The model under review builds one solid part; all positions refer to its coordinate system, in mm. A direction names the side the tool comes from. Round coordinates to 2 decimals unless told otherwise and drop trailing zeros. Loops run counter-clockwise (first coordinate to the right, second up) from the corner with the lowest first, then second, coordinate; pieces in that order, holes last. Notation, with made-up numbers: M -14.75,0 L 5.25,0 A15 cw 5.25,17 Z; hole C -25,51 d4. An arc over 180 degrees is marked long. Answer in a Markdown table with one row per item. Add a question column.
from build123d import *

# Parameters (mm, degrees)
SALIENTE_EXTRUIR1_DEPTH = 299.79
CROQUIS2_W              = 2
CROQUIS2_H              = 10
SALIENTE_EXTRUIR2_DEPTH = 134.79


with BuildPart() as part:
    # Croquis1 → Saliente-Extruir1 (new body)
    with BuildSketch(Plane.XY):
        Polygon((-6.5, 0), (6.5, 0), (10.956890061, 14.1), (40.206890061, 14.1), (40.206890061, -7.9), (-39.793109939, -7.9), (-39.793109939, 14.1), (-10.543109939, 14.1), align=None)
    extrude(amount=-SALIENTE_EXTRUIR1_DEPTH)

    # Croquis2 → Saliente-Extruir2 (add)
    with BuildSketch(Plane.XY):
        with Locations((-12.543109939, 19.1)):
            Rectangle(CROQUIS2_W, CROQUIS2_H)
    saliente_extruir2 = extrude(amount=-SALIENTE_EXTRUIR2_DEPTH)

    # Simetría1: Saliente-Extruir2 across plane
    add(saliente_extruir2.mirror(Plane(origin=(0, 0, 0), x_dir=(0, 0, 1), z_dir=(1, 0, 0))))


solid = part.part
1. Take a section at B-B, the plane z = -77.5. State the section outline as (x, y) points, and give its area (3 significant figures).
2. Take a section at D-D, the plane y = 6.5. State the section outline as (x, z) points.
3. Mouldability with a two-part tool opening along X and no side actions: class faces 4 (the flat face through (13.543, 19, -66)), 5 (the flat face through (1, -7.9, -148)), 6 (the flat face through (8.697, 6.951, -147.796)) as released by +X, released by -X, zero draft, split by the parting line, or undercut.
4. Take a section at A-A, the plane y = 18.5. State the section outline as (x, z) points.
5. Take a section at C-C, the plane x = 1. State the section outline as (y, z) points, and give its area (3 significant figures).
6. Machinability: for faces 1 (the flat face through (1, -2, 0)), 2 (the flat face through (0, 0, -148)), 3 (the flat face through (-13.543, 19, -66)), which of the approach directions +Z, -Z, +X, -X, +Y, -Y give a long, thin tool a straight path to every point of the face, cutting with its end or side? Answer none if there is none.
7. To check wall thickness, follow probe 1 along X at (y, z) = (20.5, -17); probe 2 along Y at (x, z) = (-18.5, -103.5); probe 3 along Y at (x, z) = (-6, -154). State the ranges of each line that lie inside material, in increasing order.
8. For pin 1 Ø4 at (x, z) = (-1, -153.5) entering from +Y; pin 2 Ø1.6 at (x, y) = (12.5, 20) entering from -Z; pin 3 Ø1 at (x, z) = (18, -82.5) entering from +Y; pin 4 Ø1 at (x, y) = (-6.5, 8.5) entering from +Z, all flat-tipped, find the tip position at first contact; note any pin that passes through.
Check sheet entries:
| question | item | result |
|---|---|---|
| 1 | outline | M -39.79,-7.9 L 40.21,-7.9 L 40.21,14.1 L 13.54,14.1 L 13.54,24.1 L 11.54,24.1 L 11.54,14.1 L 10.96,14.1 L 6.5,0 L -6.5,0 L -10.54,14.1 L -11.54,14.1 L -11.54,24.1 L -13.54,24.1 L -13.54,14.1 L -39.79,14.1 Z |
| 1 | area | 1,560 mm^2 |
| 2 | outline | M -39.79,-299.79 L -8.36,-299.79 L -8.36,0 L -39.79,0 Z; M 8.55,-299.79 L 40.21,-299.79 L 40.21,0 L 8.55,0 Z |
| 3 | face 4 | released by +X |
| 3 | face 5 | zero draft |
| 3 | face 6 | undercut |
| 4 | outline | M -13.54,-134.79 L -11.54,-134.79 L -11.54,0 L -13.54,0 Z; M 11.54,-134.79 L 13.54,-134.79 L 13.54,0 L 11.54,0 Z |
| 5 | outline | M -7.9,-299.79 L 0,-299.79 L 0,0 L -7.9,0 Z |
| 5 | area | 2,370 mm^2 |
| 6 | face 1 | +Z, +X, -X, +Y, -Y |
| 6 | face 2 | +Z, -Z, +Y |
| 6 | face 3 | +Z, -Z, -X, +Y |
| 7 | probe 1 | x = -13.54 to -11.54, 11.54 to 13.54 |
| 7 | probe 2 | y = -7.9 to 14.1 |
| 7 | probe 3 | y = -7.9 to 0 |
| 8 | pin 1 | stops at y = 0 |
| 8 | pin 2 | stops at z = -134.79 |
| 8 | pin 3 | stops at y = 14.1 |
| 8 | pin 4 | passes through |
